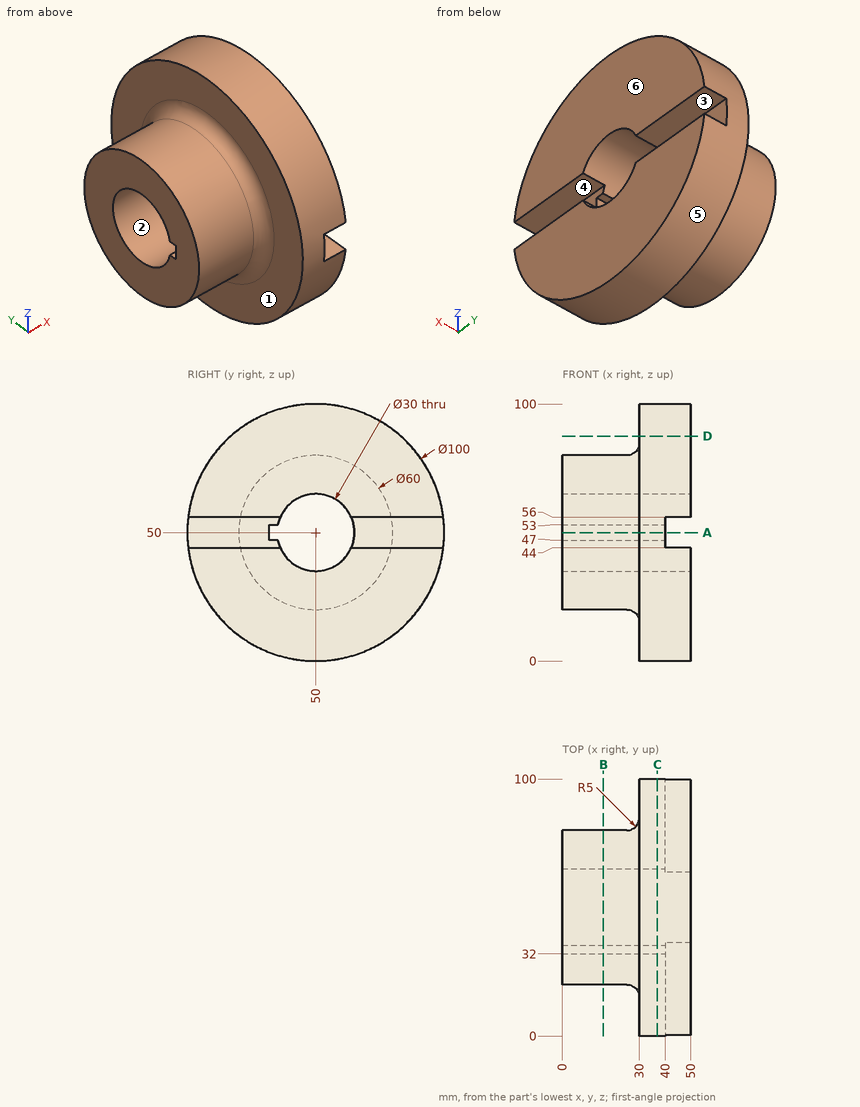
Source: three-view drawing plus pictorial views. Frame: mm from the lowest corner of the part. A direction names the side the tool comes from. Coordinates: 2 decimals unless noted, no trailing zeros. Loops run counter-clockwise (first coordinate to the right, second up) from the corner with the lowest first, then second, coordinate; pieces in that order, holes last. Notation, with made-up numbers: (24.5, 23.5) -> (47.5, 23.5) arc R24 ccw to (47.5, 48.5) -> close; hole circle Ø11 at (14.5, 12). An arc over 180 degrees is marked (long way). Answer in a Markdown table with one row per item. Add a question column.
Q1. Section C-C on x = 37. Return the cut outline in (y, z), and give its area (3 significant figures).
Q2. Pull-direction query (Z, two-part tool) for the marked faces 4, 5 and 6; classes: pulls with the +Z half, pulls with the -Z half, needs draft (parallel to the pull), parting line crosses it, or undercut.
Q3. Reachability of the marked faces 1, 2 and 3 from +Z, -Z, +X, -X, +Y, -Y: full face, straight path, thin tool, end or side. Return the list, or none.
Q4. Ray query, line 1 along Y through (x, z) = (36, 50); line 2 along Y through (x, z) = (21, 50); line 3 along X through (y, z) = (15, 72). Return the intervals inside material, ascending.
Q5. Section A-A on z = 50. Return the cut outline in (x, y).
Q6. Section B-B on x = 16. Return the cut outline in (y, z), and give its area (3 significant figures).
Q7. Contact query for flat-ended pins moving along their axis: pin 1 Ø1.7 at (x, y) = (15.5, 33.5) entering from -Z; pin 2 Ø5 at (x, y) = (47, 90) entering from +Z; pin 3 Ø3 at (x, y) = (44.5, 14.5) entering from +Z; pin 4 Ø24 at (y, z) = (50, 50) entering from +X. Output: stop coordinate, or through.
Q8. Section D-D on z = 87.5. Return the cut outline in (x, y), and give its area (3 significant figures).
Computed values:
| question | item | result |
|---|---|---|
| 1 | outline | circle Ø100 at (50, 50); hole (32, 47) -> (35.3, 47) arc R15 ccw (long way) to (35.3, 53) -> (32, 53) -> close |
| 1 | area | 7,130 mm^2 |
| 2 | face 4 | undercut |
| 2 | face 5 | parting line crosses it |
| 2 | face 6 | needs draft |
| 3 | face 1 | -X |
| 3 | face 2 | +X, -X |
| 3 | face 3 | +X, +Y, -Y |
| 4 | line 1 | y = 0 to 32, 65 to 100 |
| 4 | line 2 | y = 20 to 32, 65 to 80 |
| 4 | line 3 | x = 30 to 50 |
| 5 | outline | (0, 20) -> (25, 20) arc R5 cw to (30, 15) -> (30, 0) -> (40, 0) -> (40, 32) -> (0, 32) -> close; (0, 65) -> (40, 65) -> (40, 100) -> (30, 100) -> (30, 85) arc R5 cw to (25, 80) -> (0, 80) -> close |
| 6 | outline | circle Ø60 at (50, 50); hole (32, 47) -> (35.3, 47) arc R15 ccw (long way) to (35.3, 53) -> (32, 53) -> close |
| 6 | area | 2,100 mm^2 |
| 7 | pin 1 | stops at z = 24.41 |
| 7 | pin 2 | stops at z = 83.07 |
| 7 | pin 3 | stops at z = 86.66 |
| 7 | pin 4 | passes through |
| 8 | outline | (30, 16.93) -> (50, 16.93) -> (50, 83.07) -> (30, 83.07) -> close |
| 8 | area | 1,320 mm^2 |
